Geometry: final body of the model. Coordinates: model frame, mm. Face numbers are marked on the shaded views. A direction names the side the tool comes from. Round coordinates to 2 decimals unless told otherwise and drop trailing zeros. Loops run counter-clockwise (first coordinate to the right, second up) from the corner with the lowest first, then second, coordinate; pieces in that order, holes last. Notation, with made-up numbers: (-28, 63.25) - (-12, 63.25) arc R31 cw to (-12, 102.25) - close; hole circle Ø1 at (41, 5.5). An arc over 180 degrees is marked (long way). Return JSON: item names as keys, results as strings. Group by question number.
1. Section D-D on x = -488.5. Return loops of the section in (y, z), and give its area (3 significant figures).
2. Draft query along Y for the marked faces 4, 5 and 6. Return one class per face: +Y half, -Y half, draft (parallel to the pull), parting line (faces both ways), or undercut.
3. Material intervals for probe 1 along X at (y, z) = (96, -28); probe 2 along Y at (x, z) = (-247, -124.5); probe 3 along Z at (x, y) = (-147.5, -51), sorted ascending.
4. Section C-C on y = 55.5. Return loops of the section in (x, z), and give its area (3 significant figures).
5. First-contact query: pin 1 Ø20.5 at (x, y) = (551.5, -90.5) entering from +Z; pin 2 Ø1.5 at (x, y) = (201, 176) entering from -Z. Flat tips, straight axial feed; report the tip coordinate or a pass-through.
6. Section A-A on x = -197.5. Count the separate pieces of the cut face and the enclosed holes in it, and give its area (3 significant figures).
7. Set-up query: the marked faces 1, 2 and 3. Return all of +Z, -Z, +X, -X, +Y, -Y with unobstructed straight access to the full face (end or side cutting, diameter ignored); none if empty.
8. Section B-B on y = -267.5. Return loops of the section in (x, z).
from build123d import *

# Parameters (mm, degrees)
F0_W     = 1200
F0_H     = 145
F1_DEPTH = 22
F0_H_2   = 100
F2_W     = 145
F2_H     = 655
F2_H_2   = 145
F3_DEPTH = 22
F4_W     = 145
F4_H     = 100
F4_H_2   = 145
F5_W     = 145
F5_H     = 145
F5_H_2   = 100
F6_DEPTH = 78
F7_W     = 145
F7_H     = 100
F7_W_2   = 1055
F7_W_3   = 1200
F7_H_2   = 145
F8_DEPTH = 22
F9_SIZE  = 15


# Not quite as in the source:
# - a feature names something its author has since deleted; it is built from what else it names


with BuildPart() as f1:
    # F0 (on Top) → F1 (new body)
    with BuildSketch(Plane.XY):
        with Locations((0, 327.5)):
            Rectangle(F0_W, F0_H)
    extrude(amount=-F1_DEPTH)



with BuildPart() as f1b:
    # F0 (on Top) → F1, piece 2 (new body)
    with BuildSketch(Plane.XY):
        with Locations((0, 163.75)):
            Rectangle(F0_W, F0_H_2)
    extrude(amount=-F1_DEPTH)


with BuildPart() as f1c:
    # F0 (on Top) → F1, piece 3 (new body)
    with BuildSketch(Plane.XY):
        Rectangle(F0_W, F0_H)
    extrude(amount=-F1_DEPTH)


with BuildPart() as f1d:
    # F0 (on Top) → F1, piece 4 (new body)
    with BuildSketch(Plane.XY):
        with Locations((0, -163.75)):
            Rectangle(F0_W, F0_H_2)
    extrude(amount=-F1_DEPTH)


with BuildPart() as f1e:
    # F0 (on Top) → F1, piece 5 (new body)
    with BuildSketch(Plane.XY):
        with Locations((0, -327.5)):
            Rectangle(F0_W, F0_H)
    extrude(amount=-F1_DEPTH)


with BuildPart() as f1_1:
    add(f1.part)

    add(f1b.part)  # F3 merges F1b

    add(f1c.part)  # F3 merges F1c

    add(f1d.part)  # F3 merges F1d

    add(f1e.part)  # F3 merges F1e
    # F2 (on face) → F3 (join)
    with BuildSketch(Plane(origin=(0, 0, -22), x_dir=(1, 0, 0), z_dir=(0, 0, -1))):
        with Locations((-527.5, -72.5)):
            Rectangle(F2_W, F2_H)
        with Locations((-527.5, 327.5)):
            Rectangle(F2_W, F2_H_2)
        with Locations((0, 327.5)):
            Rectangle(F2_W, F2_H_2)
        with Locations((0, -72.5)):
            Rectangle(F2_W, F2_H)
        with Locations((527.5, 327.5)):
            Rectangle(F2_W, F2_H_2)
        with Locations((527.5, -72.5)):
            Rectangle(F2_W, F2_H)
    extrude(amount=F3_DEPTH)

    # F4 (on face) + F5 (on face) → F6 (join)
    with BuildSketch(Plane(origin=(0, 0, -44), x_dir=(1, 0, 0), z_dir=(0, 0, -1))):
        with Locations((-527.5, -350)):
            Rectangle(F4_W, F4_H)
        with Locations((-527.5, 350)):
            Rectangle(F4_W, F4_H)
        with Locations((527.5, -350)):
            Rectangle(F4_W, F4_H)
        with Locations((527.5, 0)):
            Rectangle(F4_W, F4_H_2)
        with Locations((527.5, 350)):
            Rectangle(F4_W, F4_H)
        with Locations((-527.5, 0)):
            Rectangle(F4_W, F4_H_2)
    with BuildSketch(Plane(origin=(0, 0, -44), x_dir=(1, 0, 0), z_dir=(0, 0, -1))):
        Rectangle(F5_W, F5_H)
        with Locations((0, 350)):
            Rectangle(F5_W, F5_H_2)
        with Locations((0, -350)):
            Rectangle(F5_W, F5_H_2)
    extrude(amount=F6_DEPTH)

    # F7 (on face) → F8 (join)
    with BuildSketch(Plane(origin=(0, 0, -122), x_dir=(1, 0, 0), z_dir=(0, 0, -1))):
        with Locations((-527.5, -350)):
            Rectangle(F7_W, F7_H)
        with Locations((72.5, -350)):
            Rectangle(F7_W_2, F7_H)
        Rectangle(F7_W_3, F7_H_2)
        with Locations((0, 350)):
            Rectangle(F7_W_3, F7_H)
    extrude(amount=F8_DEPTH)

    # F9
    f9_edges = [f1_1.edges().sort_by_distance(p)[0] for p in [
        (-600, -400, -72),
        (600, -400, -72),
        (600, 400, -72),
        (-600, 400, -72),
    ]]
    chamfer(f9_edges, length=F9_SIZE)


solid = f1_1.part
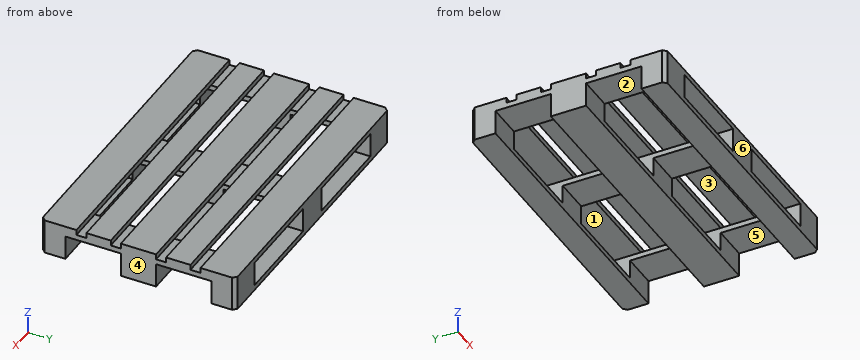
Taken from the geometry:
{
 "1": {"outline": "(-400, -144) - (-300, -144) - (-300, -44) - (-72.5, -44) - (-72.5, -144) - (72.5, -144) - (72.5, -44) - (300, -44) - (300, -144) - (400, -144) - (400, 0) - (255, 0) - (255, -22) - (213.75, -22) - (213.75, 0) - (113.75, 0) - (113.75, -22) - (72.5, -22) - (72.5, 0) - (-72.5, 0) - (-72.5, -22) - (-113.75, -22) - (-113.75, 0) - (-213.75, 0) - (-213.75, -22) - (-255, -22) - (-255, 0) - (-400, 0) - close", "area": "66,100 mm2"},
 "2": {"face 4": "draft", "face 5": "undercut", "face 6": "-Y half"},
 "3": {"probe 1": "-600 to -455, -72.5 to 72.5, 455 to 600", "probe 2": "-400 to -300, -72.5 to 72.5, 300 to 400", "probe 3": "-144 to -122, -22 to 0"},
 "4": {"outline": "(-600, -144) - (600, -144) - (600, 0) - (-600, 0) - close; hole (-455, -122) - (-72.5, -122) - (-72.5, -22) - (-455, -22) - close; hole (72.5, -122) - (455, -122) - (455, -22) - (72.5, -22) - close", "area": "96,300 mm2"},
 "5": {"pin 1": "z = -22", "pin 2": "z = -22"},
 "6": {"separate pieces": "8", "enclosed holes": "0", "area": "21,600 mm2"},
 "7": {"face 1": "+Y, -Y", "face 2": "-Z, +X, -X", "face 3": "-Z, +Y, -Y"},
 "8": {"outline": "(-600, -44) - (-455, -44) - (-455, -22) - (-72.5, -22) - (-72.5, -44) - (72.5, -44) - (72.5, -22) - (455, -22) - (455, -44) - (600, -44) - (600, 0) - (-600, 0) - close"}
}
